Geometry: final body of the model. Coordinates: model frame, mm. Face numbers are marked on the shaded views. A direction names the side the tool comes from. Round coordinates to 2 decimals unless told otherwise and drop trailing zeros. Loops run counter-clockwise (first coordinate to the right, second up) from the corner with the lowest first, then second, coordinate; pieces in that order, holes last. Notation, with made-up numbers: (-19.75, 67) - (33.25, 67) arc R27 ccw to (33.25, 90) - close; hole circle Ø7 at (32.25, -25). An arc over 180 degrees is marked (long way). Return JSON: item names as keys, results as strings. Group by question number.
1. Section B-B on y = -15.5. Return loops of the section in (x, z).
2. Section C-C on z = -1.75. Count the separate pieces of the cut face and the enclosed holes in it, and give its area (3 significant figures).
3. Material intervals for probe 1 along X at (y, z) = (-4, -1.2); probe 2 along X at (y, z) = (-6, -0.55); probe 3 along Y at (x, z) = (-2, -2.9), sorted ascending.
4. Section D-D on x = -12.5. Return loops of the section in (y, z), and give its area (3 significant figures).
5. First-contact query: pin 1 Ø4.5 at (x, y) = (28, -5) entering from +Z; pin 2 Ø5.5 at (x, y) = (-26.28, -5.66) entering from +Z; pin 3 Ø1.3 at (x, z) = (-21.5, -1) entering from -Y; pin 4 Ø1.5 at (x, y) = (-32.77, -11.48) entering from +Z. Flat tips, straight axial feed; report the tip coordinate or a pass-through.
6. Draft query along Y for the marked faces 3, 4 and 5. Return one class per face: +Y half, -Y half, draft (parallel to the pull), parting line (faces both ways), or undercut.
7. Set-up query: the marked faces 1 and 2. Return all of +Z, -Z, +X, -X, +Y, -Y with unobstructed straight access to the full face (end or side cutting, diameter ignored); none if empty.
8. Section A-A on x = -35. Return loops of the section in (y, z), and give its area (3 significant figures).
from build123d import *

# Parameters (mm, degrees)
SKETCH4_R                = 4.7244
STOCK_DEPTH              = 4.4196
SKETCH7_R                = 7.8994
CV_GEAR_WELL_DEPTH       = 4.0132
SKETCH8_R                = 2.2987
IDLER_GEAR_WELL_DEPTH    = 4.2926
SKETCH9_R                = 1.27
SKETCH9_R_2              = 4.4196
OUTDRIVE_GEAR_WELL_DEPTH = 4.4196


with BuildPart() as part:
    # Sketch4 → Stock (new body)
    with BuildSketch(Plane.XY):
        with BuildLine():
            Line((-32.450767839, 9.202272933), (-41.975767839, 9.202272933))
            ThreePointArc((-41.975767839, 9.202272933), (-44.220831869, 8.272336964), (-45.150767839, 6.027272933))
            Line((-45.150767839, 6.027272933), (-45.150767839, -3.497727067))
            ThreePointArc((-45.150767839, -3.497727067), (-44.220831869, -5.742791097), (-41.975767839, -6.672727067))
            Line((-41.975767839, -6.672727067), (-35.942804696, -6.672727067))
            Line((-35.942804696, -6.672727067), (-35.942804696, -11.480556714))
            ThreePointArc((-35.942804696, -11.480556714), (-35.012868726, -13.725620744), (-32.767804696, -14.655556714))
            Line((-32.767804696, -14.655556714), (8.354795304, -14.655556714))
            Line((8.354795304, -14.655556714), (8.354795304, -17.830556714))
            ThreePointArc((8.354795304, -17.830556714), (9.284731274, -20.075620744), (11.529795304, -21.005556714))
            Line((11.529795304, -21.005556714), (36.929795304, -21.005556714))
            ThreePointArc((36.929795304, -21.005556714), (39.174859334, -20.075620744), (40.104795304, -17.830556714))
            Line((40.104795304, -17.830556714), (40.104795304, 7.569443286))
            ThreePointArc((40.104795304, 7.569443286), (39.174859334, 9.814507317), (36.929795304, 10.744443286))
            Line((36.929795304, 10.744443286), (11.529795304, 10.744443286))
            ThreePointArc((11.529795304, 10.744443286), (9.284731274, 9.814507317), (8.354795304, 7.569443286))
            Line((8.354795304, 7.569443286), (8.354795304, 4.394443286))
            Line((8.354795304, 4.394443286), (-29.275767839, 4.394443286))
            Line((-29.275767839, 4.394443286), (-29.275767839, 6.027272933))
            ThreePointArc((-29.275767839, 6.027272933), (-30.205703809, 8.272336964), (-32.450767839, 9.202272933))
        make_face()
        with Locations((24.367264728, -5.266950247)):
            Circle(SKETCH4_R, mode=Mode.SUBTRACT)
    extrude(amount=-STOCK_DEPTH)

    # Sketch7 → CV Gear Well (cut)
    with BuildSketch(Plane(origin=(0, 0, 0), x_dir=(-1, 0, 0), z_dir=(0, 0, -1))):
        with Locations((-24.367264728, -5.266950247)):
            Circle(SKETCH7_R)
    extrude(amount=CV_GEAR_WELL_DEPTH, mode=Mode.SUBTRACT)

    # Sketch8 → Idler Gear Well (cut)
    with BuildSketch(Plane(origin=(0, 0, 0), x_dir=(-1, 0, 0), z_dir=(0, 0, -1))):
        with Locations((26.278771935, -5.664889979)):
            Circle(SKETCH8_R)
        with Locations((11.496428235, -5.54874107)):
            Circle(SKETCH8_R)
        with Locations((-3.285915465, -5.432592161)):
            Circle(SKETCH8_R)
    extrude(amount=IDLER_GEAR_WELL_DEPTH, mode=Mode.SUBTRACT)

    # Sketch9 → Outdrive Gear Well (cut)
    with BuildSketch(Plane(origin=(0, 0, 0), x_dir=(-1, 0, 0), z_dir=(0, 0, -1))):
        with Locations((32.767804696, -11.480556714)):
            Circle(SKETCH9_R)
        with Locations((-11.529795304, -17.830556714)):
            Circle(SKETCH9_R)
        with Locations((-11.529795304, 7.569443286)):
            Circle(SKETCH9_R)
        with Locations((-36.929795304, 7.569443286)):
            Circle(SKETCH9_R)
        with Locations((37.124150155, 0.645421982)):
            Circle(SKETCH9_R_2)
    extrude(amount=OUTDRIVE_GEAR_WELL_DEPTH, mode=Mode.SUBTRACT)


solid = part.part
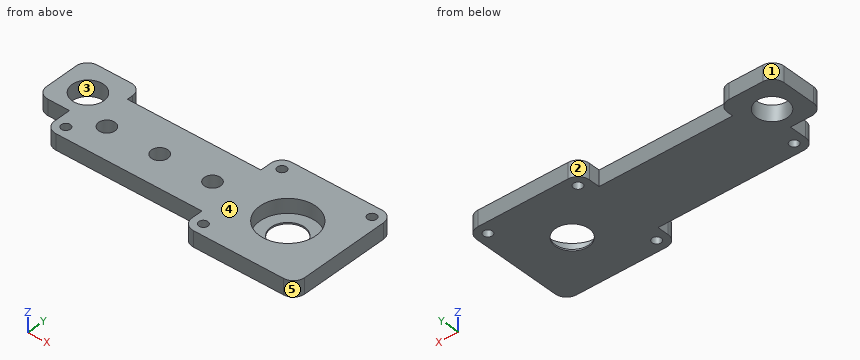
Taken from the geometry:
{
 "1": {"outline": "(8.35, -4.42) - (40.1, -4.42) - (40.1, 0) - (8.35, 0) - close"},
 "2": {"separate pieces": "1", "enclosed holes": "9", "area": "1,690 mm2"},
 "3": {"probe 1": "-45.11 to -27.86, -24.69 to -13.2, -9.8 to 1.49, 5.08 to 16.57, 32.16 to 40.1", "probe 2": "-43.93 to -28.55, -24 to -13.75, -9.24 to 1.06, 5.51 to 16.5, 32.23 to 40.1", "probe 3": "-14.66 to 4.39"},
 "4": {"outline": "(-14.66, -4.42) - (4.39, -4.42) - (4.39, 0) - (-3.48, 0) - (-3.48, -4.29) - (-7.62, -4.29) - (-7.62, 0) - (-14.66, 0) - close", "area": "66.4 mm2"},
 "5": {"pin 1": "z = -4.01", "pin 2": "z = 0", "pin 3": "y = -14.66", "pin 4": "through"},
 "6": {"face 3": "undercut", "face 4": "draft", "face 5": "-Y half"},
 "7": {"face 1": "+Z, -Z, -X, +Y", "face 2": "+Z, -Z, +Y"},
 "8": {"outline": "(-13.74, -4.42) - (-3.23, -4.42) - (-3.23, 0) - (-13.74, 0) - close; (4.52, -4.42) - (9.2, -4.42) - (9.2, 0) - (4.52, 0) - close", "area": "67.1 mm2"}
}
